```python
from build123d import *

# Parameters (mm, degrees)
F0_R        = 1.2
F0_W        = 12
F0_H        = 2.5
F0_R_2      = 1.75
F1_DEPTH    = 1.2
F2_DEPTH    = 7
F3_T1_DEPTH = 17
F3_T3_DEPTH = 16.6824583655
F3_T5_DEPTH = 11.2


# Not quite as in the source:
# - a fillet or chamfer that OpenCascade refuses, or shapes differently, is made with other operations: its cross-section is extruded or revolved along the edge and cut away or added
# - a feature names something its author has since deleted; it is built from what else it names


with BuildPart() as f1:
    # F0 (on Top) → F1 (new body)
    with BuildSketch(Plane.XY):
        Polygon((-6, -17.5), (-6, -15), (-12.5, -15), (-12.5, -19), (-6, -19), align=None)
        with Locations((-9.2, -17)):
            Circle(F0_R, mode=Mode.SUBTRACT)
        with Locations((0, -16.25)):
            Rectangle(F0_W, F0_H)
        Polygon((12.5, -19), (12.5, -15), (6, -15), (6, -17.5), (6, -19), align=None)
        with Locations((9.2, -17)):
            Circle(F0_R, mode=Mode.SUBTRACT)
        with BuildLine():
            Line((12.5, -15), (15, -15))
            Line((15, -15), (15, 0))
            Line((15, 0), (14.25, 0))
            ThreePointArc((14.25, 0), (0, -14.25), (-14.25, 0))
            Line((-14.25, 0), (-15, 0))
            Line((-15, 0), (-15, -15))
            Line((-15, -15), (-12.5, -15))
            Line((-12.5, -15), (-6, -15))
            Line((-6, -15), (6, -15))
            Line((6, -15), (12.5, -15))
        make_face()
        with Locations((-12, -12)):
            Circle(F0_R_2, mode=Mode.SUBTRACT)
        with Locations((12, -12)):
            Circle(F0_R_2, mode=Mode.SUBTRACT)
    extrude(amount=F1_DEPTH)

    # F0 (on Top) → F2 (join)
    with BuildSketch(Plane.XY):
        with Locations((0, -16.25)):
            Rectangle(F0_W, F0_H)
        Polygon((-6, -17.5), (-6, -15), (-12.5, -15), (-12.5, -19), (-6, -19), align=None)
        with Locations((-9.2, -17)):
            Circle(F0_R, mode=Mode.SUBTRACT)
        Polygon((12.5, -19), (12.5, -15), (6, -15), (6, -17.5), (6, -19), align=None)
        with Locations((9.2, -17)):
            Circle(F0_R, mode=Mode.SUBTRACT)
    extrude(amount=F2_DEPTH)

    # F3: fillet of radius 2 on 6 edges, made by hand

    # F3_s2 → F3_t1 (cut)
    with BuildSketch(Plane.XY.offset(-5)):
        with BuildLine():
            ThreePointArc((-12.5, -17), (-11.9142135624, -18.4142135624), (-10.5, -19))
            Line((-10.5, -19), (-12.5, -19))
            Line((-12.5, -19), (-12.5, -17))
        make_face()
        with BuildLine():
            ThreePointArc((10.5, -19), (11.9142135624, -18.4142135624), (12.5, -17))
            Line((12.5, -17), (12.5, -19))
            Line((12.5, -19), (10.5, -19))
        make_face()
    extrude(amount=F3_T1_DEPTH, mode=Mode.SUBTRACT)

    # F3_s4 → F3_t3 (cut)
    with BuildSketch(Plane.XY.offset(-4.8412291828)):
        with BuildLine():
            ThreePointArc((-6, -17.5), (-6.7117468017, -18.5811388301), (-7.9364916731, -19))
            Line((-7.9364916731, -19), (-6, -19))
            Line((-6, -19), (-6, -17.5))
        make_face()
        with BuildLine():
            ThreePointArc((7.9364916731, -19), (6.7117468017, -18.5811388301), (6, -17.5))
            Line((6, -17.5), (6, -19))
            Line((6, -19), (7.9364916731, -19))
        make_face()
    extrude(amount=F3_T3_DEPTH, mode=Mode.SUBTRACT)

    # F3_s6 → F3_t5 (cut)
    with BuildSketch(Plane.XY.offset(-5)):
        with BuildLine():
            ThreePointArc((15, -13), (14.4142135624, -14.4142135624), (13, -15))
            Line((13, -15), (15, -15))
            Line((15, -15), (15, -13))
        make_face()
        with BuildLine():
            ThreePointArc((-15, -13), (-14.4142135624, -14.4142135624), (-13, -15))
            Line((-13, -15), (-15, -15))
            Line((-15, -15), (-15, -13))
        make_face()
    extrude(amount=F3_T5_DEPTH, mode=Mode.SUBTRACT)


solid = f1.part
```
The model under review builds one solid part; all positions refer to its coordinate system, in mm. A direction names the side the tool comes from. Coordinates: 2 decimals unless noted, no trailing zeros. Write each loop counter-clockwise with the first axis right and the second up, starting at its lowest first coordinate (ties: lowest second). Pieces come first, ordered by that corner, then holes. Notation, with made-up numbers: (85, 67) - (111, 67) arc R34 cw to (111, 103) - close; hole circle Ø6 at (-30, -33). An arc over 180 degrees is marked (long way). Write item = value, one per line.
(1) Consider section D-D, the plane y = -8. Give the boundary of the cut face in (x, z).
Result sheet:
outline = (-15, 0) - (-11.79, 0) - (-11.79, 1.2) - (-15, 1.2) - close; (11.79, 0) - (15, 0) - (15, 1.2) - (11.79, 1.2) - close
(2) Machinability: for faces 1 (the face through (-12.5, -16, 3)), 2 (the face through (12.5, -16, 3)), 3 (the face through (-6.7, -18.57, 3.45)), which of the approach directions +Z, -Z, +X, -X, +Y, -Y give a long, thin tool a straight path to every point of the face, cutting with its end or side? Answer none if there is none.
Result sheet:
face_1 = +Z, -Z, -X, -Y
face_2 = +Z, -Z, +X, -Y
face_3 = +Z, -Z, -Y
(3) Consider section C-C, the plane x = 12. Give the boundary of the cut face in (y, z), then the cut area to 3 significant figures.
Result sheet:
outline = (-18.32, 0) - (-13.75, 0) - (-13.75, 1.2) - (-15, 1.2) - (-15, 7) - (-18.32, 7) - close; (-10.25, 0) - (-7.69, 0) - (-7.69, 1.2) - (-10.25, 1.2) - close
area = 27.8 mm^2
(4) For P1, Ø2, axis at y = -9, z = 2.5, coming from the -X side; P2, Ø1.6, axis at y = -15.5, z = 2, coming from the -X side; P3, Ø3.5, axis at x = -2, z = 3, coming from the -Y side; P4, Ø4, axis at x = 12, y = -12, coming from the +Z side, all flat-tipped, find the tip position at first contact; note any pin that passes through.
Result sheet:
P1 = through
P2 = -12.5
P3 = -17.5
P4 = 1.2
(5) Consider section A-A, the plane z = 1.75. Give the boundary of the cut face in (x, y), then the cut area to 3 significant figures.
Result sheet:
outline = (-12.5, -17) arc R2 ccw to (-10.5, -19) - (-7.94, -19) arc R2 ccw to (-6, -17.5) - (6, -17.5) arc R2 ccw to (7.94, -19) - (10.5, -19) arc R2 ccw to (12.5, -17) - (12.5, -15) - (-12.5, -15) - close; hole circle Ø2.4 at (-9.2, -17); hole circle Ø2.4 at (9.2, -17)
area = 69.7 mm^2
(6) Mouldability with a two-part tool opening along X and no side actions: class faces 4 (the face through (-11.1, -10.5, 0.6)), 5 (the face through (-9, -19, 3)), 6 (the face through (-8.646, -18.065, 3.451)), 7 (the face through (14.43, -14.4, 0.59)) as pulls with the +X half, pulls with the -X half, needs draft (parallel to the pull), parting line crosses it, or undercut.
Result sheet:
face_4 = undercut
face_5 = needs draft
face_6 = undercut
face_7 = pulls with the +X half
(7) For line 1 (X direction, y = -16.5, z = 6.5); line 2 (Y direction, x = 9.2, z = 3.25); line 3 (X direction, y = -15.5, z = 6), list the stretches that pass through material, from the lowest coordinate up. Write a range as [from, to].
Result sheet:
line_1 = [-12.5, -10.29], [-8.11, 8.11], [10.29, 12.5]
line_2 = [-19, -18.2], [-15.8, -15]
line_3 = [-12.5, 12.5]
(8) Consider section B-B, the plane y = -12. Give the boundary of the cut face in (x, z), then the cut area to 3 significant figures.
Result sheet:
outline = (-15, 0) - (-13.75, 0) - (-13.75, 1.2) - (-15, 1.2) - close; (-10.25, 0) - (-7.69, 0) - (-7.69, 1.2) - (-10.25, 1.2) - close; (7.69, 0) - (10.25, 0) - (10.25, 1.2) - (7.69, 1.2) - close; (13.75, 0) - (15, 0) - (15, 1.2) - (13.75, 1.2) - close
area = 9.16 mm^2
